Geometry: final body of the model. Coordinates: model frame, mm. A direction names the side the tool comes from. Round coordinates to 2 decimals unless told otherwise and drop trailing zeros. Loops run counter-clockwise (first coordinate to the right, second up) from the corner with the lowest first, then second, coordinate; pieces in that order, holes last. Notation, with made-up numbers: M 25.25,48.5 L 29.25,48.5 A22 cw 29.25,60.5 Z; hole C 89.5,21 d1. An arc over 180 degrees is marked long. Answer as a JSON object with one key per item and string values.
Autodesk Inventor part; units mm, degrees
ref_plane "YZ Plane" through (0, 0, 0) normal (1, 0, 0) x (0, 1, 0)
ref_plane "XZ Plane" through (0, 0, 0) normal (0, 1, 0) x (-1, 0, 0)
ref_plane "XY Plane" through (0, 0, 0) normal (0, 0, 1) x (1, 0, 0)
sketch "Skizze3" plane through (0, 0, 0) normal (0, 0, 1) x (1, 0, 0)
  line L0 (0, 0) -> (-30, 0)
  line L1 (-30, 0) -> (-30, 80)
  line L2 (-30, 80) -> (0, 80)
  line L3 (0, 80) -> (0, 0)
  line L4 (-30, 78.2) -> (-35.85, 78.2)
  line L5 (-35.85, 78.2) -> (-35.85, 40)
  line L6 (-35.85, 40) -> (-30, 40)
  line L7 (-30, 40) -> (-30, 78.2)
  line L8 (-30, 80) -> (-15, 80)
  line L9 (-15, 80) -> (-15, 85.85)
  line L10 (-15, 85.85) -> (-30, 85.85)
  line L11 (-30, 85.85) -> (-30, 80)
  point P0 (-30, 40)
  point P1 (-15, 80)
  dimension "d4" = 80
  dimension "d5" = 30
  dimension "d6" = 5.85
  dimension "d7" = 5.85
  dimension "d8" = 1.8
extrude "Extrusion3" add sketch "Skizze3" along normal blind 5 contours L0 L1 L2 L3
extrude "Extrusion4" add sketch "Skizze3" along normal blind 5 contours L6 L5 L4 L1 | L2 L11 L10 L9
fillet "Rundung1" radius 2 2 edges at (-35.85, 78.2, 2.5) (-30, 85.85, 2.5)
mirror "Spiegeln1" about plane through (-15, 80, 0) normal (1, 0, 0) of "Extrusion4", "Rundung1"
mirror "Spiegeln2" about plane through (5.85, 40, 0) normal (0, -1, 0) of "Extrusion4", "Rundung1", "Spiegeln1"
fillet "Rundung2" radius 1.5 4 edges at (0, 78.2, 2.5) (-30, 78.2, 2.5) (-30, 1.8, 2.5) (0, 1.8, 2.5)
equation "\"d7\" = d6"
properties part number "BT705_trajan20_21" material "Acryl"
1) Cut plane A-A on z = 0.85. Return the cut outline in (x, y).
Geometry results:
{"outline": "M -35.85,3.8 A2 ccw -33.85,1.8 L -31.5,1.8 A1.5 cw -30,0.3 L -30,-3.85 A2 ccw -28,-5.85 L -2,-5.85 A2 ccw 0,-3.85 L 0,0.3 A1.5 cw 1.5,1.8 L 3.85,1.8 A2 ccw 5.85,3.8 L 5.85,76.2 A2 ccw 3.85,78.2 L 1.5,78.2 A1.5 cw 0,79.7 L 0,83.85 A2 ccw -2,85.85 L -28,85.85 A2 ccw -30,83.85 L -30,79.7 A1.5 cw -31.5,78.2 L -33.85,78.2 A2 ccw -35.85,76.2 Z"}
2) Set-up query: faces 4 (the face through (-30, -2, 2)), 5 (the face through (-30, 82, 2)), 6 (the face through (-35.85, 41, 2)), 7 (the face through (0, 82, 2)), 8 (the face through (0, -2, 2)). Return all of +Z, -Z, +X, -X, +Y, -Y with unobstructed straight access to the full face (end or side cutting, diameter ignored); none if empty.
Geometry results:
{"face 4": "+Z, -Z, -X, -Y", "face 5": "+Z, -Z, -X, +Y", "face 6": "+Z, -Z, -X, +Y, -Y", "face 7": "+Z, -Z, +X, +Y", "face 8": "+Z, -Z, +X, -Y"}
3) Pull-direction query (Z, two-part tool) for faces 1 (the face through (-33, 1.8, 2)), 2 (the face through (-15, 41, 0)), 3 (the face through (-15, 41, 5)); classes: +Z half, -Z half, draft (parallel to the pull), parting line (faces both ways), or undercut.
Geometry results:
{"face 1": "draft", "face 2": "-Z half", "face 3": "+Z half"}
4) Line query: probe 1 along X at (y, z) = (81.5, 1.65); probe 2 along Y at (x, z) = (-32.5, 1.45); probe 3 along Y at (x, z) = (-1.5, 4.1). Output: solid intervals per line, ascending.
Geometry results:
{"probe 1": "-30 to 0", "probe 2": "1.8 to 78.2", "probe 3": "-5.79 to 85.79"}
5) First-contact query: pin 1 (0.7 mm diameter, centred on x = 3, z = 1.5, fed in from +Y); pin 2 (1.9 mm diameter, centred on x = -33, z = 1.5, fed in from -Y); pin 3 (3 mm diameter, centred on x = 0.5, z = 2.5, fed in from -Y). Flat tips, straight axial feed; report the tip coordinate or a pass-through.
Geometry results:
{"pin 1": "y = 78.2", "pin 2": "y = 1.8", "pin 3": "y = -5.58"}
